```python
from build123d import *

# Parameters (mm, degrees)
ESQUISSE1_W        = 200
ESQUISSE1_H        = 300
ESQUISSE1_R        = 1.5
ESQUISSE1_R_2      = 3
BOSS_EXTRU_1_DEPTH = 1


with BuildPart() as part:
    # Esquisse1 → Boss.-Extru.1 (new body)
    with BuildSketch(Plane(origin=(0, 0, 0), x_dir=(1, 0, 0), z_dir=(0, 1, 0))):
        Rectangle(ESQUISSE1_W, ESQUISSE1_H)
        with Locations((-37.5, -45)):
            Circle(ESQUISSE1_R, mode=Mode.SUBTRACT)
        with Locations((-7.5, -45)):
            Circle(ESQUISSE1_R, mode=Mode.SUBTRACT)
        with Locations((-37.5, -10)):
            Circle(ESQUISSE1_R, mode=Mode.SUBTRACT)
        with Locations((37.5, 10)):
            Circle(ESQUISSE1_R, mode=Mode.SUBTRACT)
        with Locations((37.5, 45)):
            Circle(ESQUISSE1_R, mode=Mode.SUBTRACT)
        with Locations((7.5, 45)):
            Circle(ESQUISSE1_R, mode=Mode.SUBTRACT)
        with Locations((85, 130)):
            Circle(ESQUISSE1_R_2, mode=Mode.SUBTRACT)
        with Locations((-85, 130)):
            Circle(ESQUISSE1_R_2, mode=Mode.SUBTRACT)
        with Locations((85, -130)):
            Circle(ESQUISSE1_R_2, mode=Mode.SUBTRACT)
        with Locations((-85, -130)):
            Circle(ESQUISSE1_R_2, mode=Mode.SUBTRACT)
        with Locations((-55, 40)):
            Circle(ESQUISSE1_R, mode=Mode.SUBTRACT)
        with Locations((-55, 58)):
            Circle(ESQUISSE1_R, mode=Mode.SUBTRACT)
        with Locations((-55, -58)):
            Circle(ESQUISSE1_R, mode=Mode.SUBTRACT)
        with Locations((-55, -40)):
            Circle(ESQUISSE1_R, mode=Mode.SUBTRACT)
        with Locations((-85, -90)):
            Circle(ESQUISSE1_R, mode=Mode.SUBTRACT)
        with Locations((-55, -90)):
            Circle(ESQUISSE1_R, mode=Mode.SUBTRACT)
        with Locations((85, -90)):
            Circle(ESQUISSE1_R, mode=Mode.SUBTRACT)
        with Locations((55, -90)):
            Circle(ESQUISSE1_R, mode=Mode.SUBTRACT)
        with Locations((55, 90)):
            Circle(ESQUISSE1_R, mode=Mode.SUBTRACT)
        with Locations((85, 90)):
            Circle(ESQUISSE1_R, mode=Mode.SUBTRACT)
        with Locations((-55, 90)):
            Circle(ESQUISSE1_R, mode=Mode.SUBTRACT)
        with Locations((-85, 90)):
            Circle(ESQUISSE1_R, mode=Mode.SUBTRACT)
        with BuildLine():
            Line((-6, -53.175), (46, -53.175))
            ThreePointArc((46, -53.175), (47.414213562, -53.760786438), (48, -55.175))
            Line((48, -55.175), (48, -77.175))
            ThreePointArc((48, -77.175), (47.414213562, -78.589213562), (46, -79.175))
            Line((46, -79.175), (-6, -79.175))
            ThreePointArc((-6, -79.175), (-7.414213562, -78.589213562), (-8, -77.175))
            Line((-8, -77.175), (-8, -55.175))
            ThreePointArc((-8, -55.175), (-7.414213562, -53.760786438), (-6, -53.175))
        make_face(mode=Mode.SUBTRACT)
        with BuildLine():
            Line((-46, 79.175), (6, 79.175))
            ThreePointArc((6, 79.175), (7.414213562, 78.589213562), (8, 77.175))
            Line((8, 77.175), (8, 55.175))
            ThreePointArc((8, 55.175), (7.414213562, 53.760786438), (6, 53.175))
            Line((6, 53.175), (-46, 53.175))
            ThreePointArc((-46, 53.175), (-47.414213562, 53.760786438), (-48, 55.175))
            Line((-48, 55.175), (-48, 77.175))
            ThreePointArc((-48, 77.175), (-47.414213562, 78.589213562), (-46, 79.175))
        make_face(mode=Mode.SUBTRACT)
        with BuildLine():
            Line((-53, -139.5000508), (53, -139.5000508))
            ThreePointArc((53, -139.5000508), (54.414213562, -138.914264362), (55, -137.5000508))
            Line((55, -137.5000508), (55, -130.772848254))
            ThreePointArc((55, -130.772848254), (54.414213562, -129.358634692), (53, -128.772848254))
            Line((53, -128.772848254), (-53, -128.772848254))
            ThreePointArc((-53, -128.772848254), (-54.414213562, -129.358634692), (-55, -130.772848254))
            Line((-55, -130.772848254), (-55, -137.5000508))
            ThreePointArc((-55, -137.5000508), (-54.414213562, -138.914264362), (-53, -139.5000508))
        make_face(mode=Mode.SUBTRACT)
        with BuildLine():
            Line((-55, 137.5000508), (-55, 130.772848254))
            ThreePointArc((-55, 130.772848254), (-54.414213562, 129.358634692), (-53, 128.772848254))
            Line((-53, 128.772848254), (53, 128.772848254))
            ThreePointArc((53, 128.772848254), (54.414213562, 129.358634692), (55, 130.772848254))
            Line((55, 130.772848254), (55, 137.5000508))
            ThreePointArc((55, 137.5000508), (54.414213562, 138.914264362), (53, 139.5000508))
            Line((53, 139.5000508), (-53, 139.5000508))
            ThreePointArc((-53, 139.5000508), (-54.414213562, 138.914264362), (-55, 137.5000508))
        make_face(mode=Mode.SUBTRACT)
    extrude(amount=BOSS_EXTRU_1_DEPTH)


solid = part.part
```
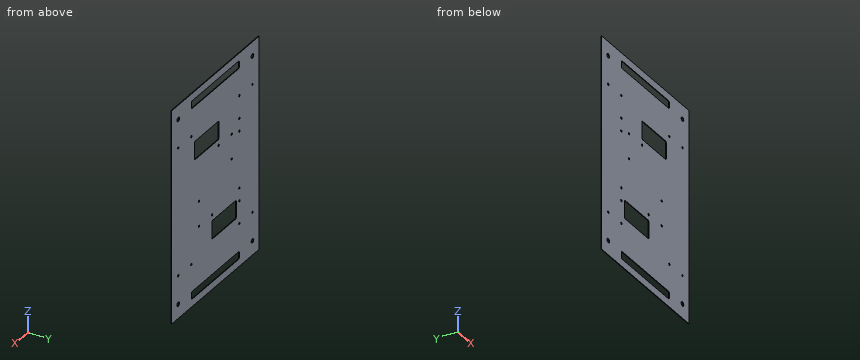
Geometry: final body of the model. Coordinates: model frame, mm. Coordinates: 2 decimals unless noted, no trailing zeros. Order: outer loops, then holes, each group sorted by start corner. A loop starts at its lowest first (then second) coordinate and runs counter-clockwise, first axis right, second up.
Item 1: Section query A-A (x = -33). Output: boundary loops of the cut face in (y, z) (3 decimals).
Answer:
outline: (0, -150) - (1, -150) - (1, -139.5) - (0, -139.5) - close; (0, -128.773) - (1, -128.773) - (1, -79.175) - (0, -79.175) - close; (0, -53.175) - (1, -53.175) - (1, 128.773) - (0, 128.773) - close; (0, 139.5) - (1, 139.5) - (1, 150) - (0, 150) - close
Item 2: Contact query for a flat-ended pin moving along its axis: P1, Ø3.5, axis at x = -55, z = 40, coming from the +Y side. Output: stop coordinate, or through.
Answer:
P1: stops at y = 1
Item 3: Material intervals for line 1 along Z through (x, y) = (-85, 0.45); line 2 along X through (y, z) = (0.55, -58); line 3 along Z through (x, y) = (-5, 0.7) (3 decimals), sorted ascending.
Answer:
line 1: z = -150 to -133, -127 to -91.5, -88.5 to 88.5, 91.5 to 127, 133 to 150
line 2: x = -100 to -56.5, -53.5 to -48, 8 to 100
line 3: z = -150 to -139.5, -128.773 to -79.175, -53.175 to 53.175, 79.175 to 128.773, 139.5 to 150
Item 4: Section query C-C (y = 0.5). State how many separate pieces and enclosed holes the cut face has, then the cut area to 3 significant figures.
Answer:
separate pieces: 1
enclosed holes: 26
area: 54,500 mm2
Item 5: Section query B-B (z = 71). Output: boundary loops of the cut face in (x, y), then the cut area to 3 significant figures.
Answer:
outline: (-100, 0) - (-8, 0) - (-8, 1) - (-100, 1) - close; (48, 0) - (100, 0) - (100, 1) - (48, 1) - close
area: 144 mm2
